The model under review builds one solid part; all positions refer to its coordinate system, in mm. A direction names the side the tool comes from. Coordinates: 2 decimals unless noted, no trailing zeros. Loops run counter-clockwise (first coordinate to the right, second up) from the corner with the lowest first, then second, coordinate; pieces in that order, holes last. Notation, with made-up numbers: M -32.75,-2.75 L -23.75,-2.75 A19 ccw -23.75,1.25 Z; hole C 39.25,21 d9. An arc over 180 degrees is marked long. Write item = value, one per line. Start each with the question number.
Q1. We need section A-A on z = -17. Give the boundary of the cut face in (x, y).
Q2. Mouldability with a two-part tool opening along Z and no side actions: class faces 4 (the face through (-8.941, 22, -7)), 5 (the face through (-17, 12.7, 16)) as released by +Z, released by -Z, zero draft, split by the parting line, or undercut.
Q3. For faces 1 (the face through (58, 12.7, 16)), 2 (the face through (-16.114, 15, -28)), 3 (the face through (-13, 33.02, -66)), list the 3-axis set-ups (+Z, -Z, +X, -X, +Y, -Y) from which the entire face can be reached by the end or side of a thin tool; tool diameter is ignored.
Q4. Clearance check with flat-ended pins moving along their axes: pin 1 Ø0.8 at (x, z) = (-12, -23) entering from +Y; pin 2 Ø4 at (y, z) = (20.5, -1.5) entering from +X; pin 3 Ø4 at (y, z) = (21.5, -28) entering from -X. State where each tip first meets the part, or that it passes through.
Q5. We need section B-B on x = 16. Give the boundary of the cut face in (y, z), and give its area (3 significant figures).
Q6. Wall thickness on probe 1 along Z at (x, y) = (6.5, 7); probe 2 along X at (y, z) = (10.35, 59.69); probe 3 along Z at (x, y) = (-4.5, 17.5): over which ranges is each line inside the solid? List them lowest first.
from build123d import *

# Parameters (mm, degrees)
SKETCH1_W            = 152.4
SKETCH1_H            = 152.4
BOSS_EXTRUDE1_DEPTH  = 5.08
SKETCH6_R            = 3.81
BOSS_EXTRUDE3_DEPTH  = 7.62
SKETCH7_W            = 152.4
SKETCH7_H            = 152.4
SKETCH7_W_2          = 139.7
SKETCH7_H_2          = 139.7
BOSS_EXTRUDE4_DEPTH  = 7.62
SKETCH9_R            = 3.81
BOSS_EXTRUDE6_DEPTH  = 27.94
SKETCH11_W           = 85.963722039
SKETCH11_H           = 81.851496928
BOSS_EXTRUDE9_DEPTH  = 20.32
SKETCH12_W           = 61.01453669
SKETCH12_H           = 25.385301209
SKETCH12_H_2         = 35.074856928
CUT_EXTRUDE1_DEPTH   = 20.32
SKETCH14_W           = 46.335678953
SKETCH14_H           = 46.77664
CUT_EXTRUDE2_DEPTH   = 7.62
SKETCH15_R           = 1.524
CUT_EXTRUDE3_DEPTH   = 3.81
SKETCH16_R           = 1.524
CUT_EXTRUDE4_DEPTH   = 3.81
BOSS_EXTRUDE10_START = -12.7
SKETCH18_W           = 165.1
SKETCH18_H           = 165.1
SKETCH18_W_2         = 152.4
SKETCH18_H_2         = 152.4
BOSS_EXTRUDE10_DEPTH = 12.7
SKETCH22_W           = 195.571726543
SKETCH22_H           = 199.98311887
SKETCH22_W_2         = 152.4
SKETCH22_H_2         = 152.4
CUT_EXTRUDE5_DEPTH   = 13.7
SKETCH24_W           = 21.59
SKETCH24_H           = 152.4
CUT_EXTRUDE6_DEPTH   = 13.7
SKETCH25_W           = 6.35
SKETCH25_H           = 139.7
BOSS_EXTRUDE11_DEPTH = 7.62
SKETCH26_W           = 3.556
SKETCH26_H           = 81.851496928
CUT_EXTRUDE7_DEPTH   = 7.62
BOSS_EXTRUDE12_START = -15.24
SKETCH28_R           = 3.81
SKETCH28_R_2         = 1.27
BOSS_EXTRUDE12_DEPTH = 15.24
CUT_EXTRUDE8_DEPTH   = 15.24


with BuildPart() as part:
    # Sketch1 → Boss-Extrude1 (new body)
    with BuildSketch(Plane(origin=(0, 0, 0), x_dir=(1, 0, 0), z_dir=(0, 1, 0))):
        Rectangle(SKETCH1_W, SKETCH1_H)
    extrude(amount=BOSS_EXTRUDE1_DEPTH)

    # Sketch6 → Boss-Extrude3 (add)
    with BuildSketch(Plane(origin=(0, 5.08, 0), x_dir=(1, 0, 0), z_dir=(0, 1, 0))):
        with Locations((62.26048, -64.77)):
            Circle(SKETCH6_R)
        with Locations((-20.21078, -64.77)):
            Circle(SKETCH6_R)
        with Locations((31.81096, -59.69)):
            Circle(SKETCH6_R)
        with Locations((31.81096, -31.78048)):
            Circle(SKETCH6_R)
        with Locations((55.90032, -16.55064)):
            Circle(SKETCH6_R)
        with Locations((-18.97888, -16.55064)):
            Circle(SKETCH6_R)
    extrude(amount=BOSS_EXTRUDE3_DEPTH)

    # Sketch7 → Boss-Extrude4 (add)
    with BuildSketch(Plane(origin=(0, 5.08, 0), x_dir=(1, 0, 0), z_dir=(0, 1, 0))):
        Rectangle(SKETCH7_W, SKETCH7_H)
        Rectangle(SKETCH7_W_2, SKETCH7_H_2, mode=Mode.SUBTRACT)
    extrude(amount=BOSS_EXTRUDE4_DEPTH)

    # Sketch9 → Boss-Extrude6 (add)
    with BuildSketch(Plane(origin=(0, 5.08, 0), x_dir=(1, 0, 0), z_dir=(0, 1, 0))):
        with Locations((63.5, -8.93064)):
            Circle(SKETCH9_R)
        with Locations((-11.7348, -8.93064)):
            Circle(SKETCH9_R)
        with Locations((63.5, 23.07336)):
            Circle(SKETCH9_R)
        with Locations((-11.7348, 23.07336)):
            Circle(SKETCH9_R)
        with Locations((-11.7348, 33.23336)):
            Circle(SKETCH9_R)
        with Locations((63.5, 33.23336)):
            Circle(SKETCH9_R)
        with Locations((63.5, 65.23736)):
            Circle(SKETCH9_R)
        with Locations((-11.7348, 65.23736)):
            Circle(SKETCH9_R)
    extrude(amount=BOSS_EXTRUDE6_DEPTH)

    # Sketch11 → Boss-Extrude9 (add)
    with BuildSketch(Plane(origin=(0, 5.08, 0), x_dir=(1, 0, 0), z_dir=(0, 1, 0))):
        with Locations((26.868138981, 28.924251536)):
            Rectangle(SKETCH11_W, SKETCH11_H)
    extrude(amount=BOSS_EXTRUDE9_DEPTH)

    # Sketch12 → Cut-Extrude1 (cut)
    with BuildSketch(Plane(origin=(0, 25.4, 0), x_dir=(1, 0, 0), z_dir=(0, 1, 0))):
        with Locations((25.122468345, 46.622124643)):
            Rectangle(SKETCH12_W, SKETCH12_H)
        with Locations((25.122468345, 5.535931536)):
            Rectangle(SKETCH12_W, SKETCH12_H_2)
    extrude(amount=-CUT_EXTRUDE1_DEPTH, mode=Mode.SUBTRACT)

    # Sketch14 → Cut-Extrude2 (cut)
    with BuildSketch(Plane(origin=(0, 25.4, 0), x_dir=(1, 0, 0), z_dir=(0, 1, 0))):
        with Locations((17.783039477, 46.46168)):
            Rectangle(SKETCH14_W, SKETCH14_H)
    extrude(amount=-CUT_EXTRUDE2_DEPTH, mode=Mode.SUBTRACT)

    # Sketch15 → Cut-Extrude3 (cut)
    with BuildSketch(Plane(origin=(0, 12.7, 0), x_dir=(1, 0, 0), z_dir=(0, 1, 0))):
        with Locations((-18.97888, -16.55064)):
            Circle(SKETCH15_R)
        with Locations((31.81096, -31.78048)):
            Circle(SKETCH15_R)
        with Locations((55.90032, -16.55064)):
            Circle(SKETCH15_R)
        with Locations((62.26048, -64.77)):
            Circle(SKETCH15_R)
        with Locations((31.81096, -59.69)):
            Circle(SKETCH15_R)
        with Locations((-20.21078, -64.77)):
            Circle(SKETCH15_R)
    extrude(amount=-CUT_EXTRUDE3_DEPTH, mode=Mode.SUBTRACT)

    # Sketch16 → Cut-Extrude4 (cut)
    with BuildSketch(Plane(origin=(0, 33.02, 0), x_dir=(1, 0, 0), z_dir=(0, 1, 0))):
        with Locations((63.5, 65.23736)):
            Circle(SKETCH16_R)
        with Locations((63.5, 33.23336)):
            Circle(SKETCH16_R)
        with Locations((63.5, 23.07336)):
            Circle(SKETCH16_R)
        with Locations((63.5, -8.93064)):
            Circle(SKETCH16_R)
        with Locations((-11.7348, -8.93064)):
            Circle(SKETCH16_R)
        with Locations((-11.7348, 23.07336)):
            Circle(SKETCH16_R)
        with Locations((-11.7348, 33.23336)):
            Circle(SKETCH16_R)
        with Locations((-11.7348, 65.23736)):
            Circle(SKETCH16_R)
    extrude(amount=-CUT_EXTRUDE4_DEPTH, mode=Mode.SUBTRACT)

    # Sketch18 → Boss-Extrude10 (add)
    with BuildSketch(Plane.XZ.offset(BOSS_EXTRUDE10_START)):
        Rectangle(SKETCH18_W, SKETCH18_H)
        Rectangle(SKETCH18_W_2, SKETCH18_H_2, mode=Mode.SUBTRACT)
    extrude(amount=BOSS_EXTRUDE10_DEPTH)

    # Sketch22 → Cut-Extrude5 (cut, through all)
    with BuildSketch(Plane(origin=(0, 12.7, 0), x_dir=(1, 0, 0), z_dir=(0, 1, 0))):
        with Locations((-3.578752524, -2.666785406)):
            Rectangle(SKETCH22_W, SKETCH22_H)
        Rectangle(SKETCH22_W_2, SKETCH22_H_2, mode=Mode.SUBTRACT)
    extrude(amount=-CUT_EXTRUDE5_DEPTH, mode=Mode.SUBTRACT)

    # Sketch24 → Cut-Extrude6 (cut, through all)
    with BuildSketch(Plane(origin=(0, 12.7, 0), x_dir=(1, 0, 0), z_dir=(0, 1, 0))):
        with Locations((-65.405, 0)):
            Rectangle(SKETCH24_W, SKETCH24_H)
    extrude(amount=-CUT_EXTRUDE6_DEPTH, mode=Mode.SUBTRACT)

    # Sketch25 → Boss-Extrude11 (add)
    with BuildSketch(Plane(origin=(0, 5.08, 0), x_dir=(1, 0, 0), z_dir=(0, 1, 0))):
        with Locations((-51.435, 0)):
            Rectangle(SKETCH25_W, SKETCH25_H)
    extrude(amount=BOSS_EXTRUDE11_DEPTH)

    # Sketch26 → Cut-Extrude7 (cut)
    with BuildSketch(Plane(origin=(0, 25.4, 0), x_dir=(1, 0, 0), z_dir=(0, 1, 0))):
        with Locations((-7.1628, 28.924251536)):
            Rectangle(SKETCH26_W, SKETCH26_H)
    extrude(amount=-CUT_EXTRUDE7_DEPTH, mode=Mode.SUBTRACT)

    # Sketch28 → Boss-Extrude12 (add)
    with BuildSketch(Plane(origin=(0, 33.02, 0), x_dir=(1, 0, 0), z_dir=(0, 1, 0)).offset(BOSS_EXTRUDE12_START)):
        with Locations((-11.7348, 65.23736)):
            Circle(SKETCH28_R)
        with Locations((-11.7348, 65.23736)):
            Circle(SKETCH28_R_2, mode=Mode.SUBTRACT)
        with Locations((-11.7348, 33.23336)):
            Circle(SKETCH28_R)
        with Locations((-11.7348, 33.23336)):
            Circle(SKETCH28_R_2, mode=Mode.SUBTRACT)
        with Locations((-11.7348, 23.07336)):
            Circle(SKETCH28_R)
        with Locations((-11.7348, 23.07336)):
            Circle(SKETCH28_R_2, mode=Mode.SUBTRACT)
        with Locations((-11.7348, -8.93064)):
            Circle(SKETCH28_R)
        with Locations((-11.7348, -8.93064)):
            Circle(SKETCH28_R_2, mode=Mode.SUBTRACT)
    extrude(amount=BOSS_EXTRUDE12_DEPTH)

    # Sketch29 → Cut-Extrude8 (cut)
    with BuildSketch(Plane(origin=(0, 33.02, 0), x_dir=(1, 0, 0), z_dir=(0, 1, 0))):
        with BuildLine():
            Line((-8.9408, -12.001496928), (-8.9408, -11.520941913))
            ThreePointArc((-8.9408, -11.520941913), (-9.198790453, -11.774010461), (-9.479597631, -12.001496928))
            Line((-9.479597631, -12.001496928), (-8.9408, -12.001496928))
        make_face()
    extrude(amount=-CUT_EXTRUDE8_DEPTH, mode=Mode.SUBTRACT)


solid = part.part
Returned:
q1.outline = M -54.61,0 L 76.2,0 L 76.2,12.7 L 69.85,12.7 L 69.85,25.4 L 55.63,25.4 L 55.63,5.08 L -5.38,5.08 L -5.38,17.78 L -8.94,17.78 L -8.94,25.4 L -16.11,25.4 L -16.11,5.08 L -48.26,5.08 L -48.26,12.7 L -54.61,12.7 Z
q2.face_4 = undercut
q2.face_5 = zero draft
q3.face_1 = +Z, +X, -X, +Y
q3.face_2 = +Y
q3.face_3 = +Z, -Z, +X, -X, +Y
q4.pin_1 = 29.21
q4.pin_2 = 69.85
q4.pin_3 = -16.11
q5.outline = M 0,-76.2 L 12.7,-76.2 L 12.7,-69.85 L 17.78,-69.85 L 17.78,-59.31 L 5.08,-59.31 L 5.08,-33.93 L 17.78,-33.93 L 17.78,-23.07 L 5.08,-23.07 L 5.08,69.85 L 12.7,69.85 L 12.7,76.2 L 0,76.2 Z
q5.area = 1,140 mm^2
q6.probe_1 = -76.2 to -59.31, -33.93 to -23.07, 69.85 to 76.2
q6.probe_2 = -54.61 to -48.26, 28 to 30.29, 33.33 to 35.62, 69.85 to 76.2
q6.probe_3 = -69.85 to -59.31, -33.93 to -23.07
